Autodesk Inventor part; units mm, degrees
ref_plane "Work Plane2" through (-10, -25.15, 0) normal (0, 1, 0) x (1, 0, 0)
ref_plane "YZ Plane" through (0, 0, 0) normal (1, 0, 0) x (0, 1, 0)
ref_plane "XZ Plane" through (0, 0, 0) normal (0, 1, 0) x (-1, 0, 0)
sketch "Sketch1" plane through (0, 0, 0) normal (0, 0, 1) x (1, 0, 0)
  line L0 (-40, 5) -> (0, 5)
  line L1 (0, 5) -> (0, -5)
  line L2 (0, -5) -> (-40, -5)
  line L3 (-40, -5) -> (-40, 5)
  line L4 (-10, 35) -> (0, 35)
  line L5 (0, 35) -> (0, 5)
  line L6 (0, 5) -> (-10, 5)
  line L7 (-10, 5) -> (-10, 35)
  point P0 (0, 0)
  point P1 (0, 5)
  dimension "d0" = 10
  dimension "d1" = 40
  dimension "d2" = 40
extrude "Extrusion1" add sketch "Sketch1" along normal blind 20
sketch "Sketch2" plane through (-10, 5, 0) normal (-1, 0, 0) x (0, 0, 1)
  line L0 (8.5, 20) -> (11.5, 20) construction
  line L1 (8.5, 17) -> (11.5, 17)
  line L2 (11.5, 23) -> (8.5, 23)
  arc A0 (8.5, 23) -> (8.5, 17) centre (8.5, 20) ccw
  arc A1 (11.5, 17) -> (11.5, 23) centre (11.5, 20) ccw
  line L3 (0, 30) -> (0, 0)
  line L4 (0, 30) -> (20, 30)
  line L5 (10, 21.547) -> (10, 15) construction
  line L6 (11.5, 20) -> (8.5, 20) construction
  line L7 (11.5, 17) -> (8.5, 17)
  line L8 (8.5, 23) -> (11.5, 23)
  arc A2 (11.5, 17) -> (11.5, 23) centre (11.5, 20) ccw
  arc A3 (8.5, 23) -> (8.5, 17) centre (8.5, 20) ccw
  point P0 (0, -5)
  point P1 (10, 20)
  point P2 (10, 18.2735)
  point P3 (10, 30)
  point P4 (10, 20)
  dimension "d5" = 6
  dimension "d6" = 3
  dimension "d7" = 10
  dimension "d8" = 10
extrude "Extrusion2" cut sketch "Sketch2" against normal through all
sketch "Sketch3" plane through (-40, 5, 0) normal (0, 1, 0) x (1, 0, 0)
  line L0 (10, -8.5) -> (10, -11.5) construction
  line L1 (7, -8.5) -> (7, -11.5)
  line L2 (13, -11.5) -> (13, -8.5)
  arc A0 (13, -8.5) -> (7, -8.5) centre (10, -8.5) ccw
  arc A1 (7, -11.5) -> (13, -11.5) centre (10, -11.5) ccw
  line L3 (30, 0) -> (0, 0)
  line L4 (0, 0) -> (0, -20)
  line L5 (15.2557, -10) -> (9.287, -10) construction
  line L6 (10, -11.5) -> (10, -8.5) construction
  line L7 (7, -11.5) -> (7, -8.5)
  line L8 (13, -8.5) -> (13, -11.5)
  arc A2 (7, -11.5) -> (13, -11.5) centre (10, -11.5) ccw
  arc A3 (13, -8.5) -> (7, -8.5) centre (10, -8.5) ccw
  point P0 (40, 0)
  point P1 (10, -10)
  point P2 (12.2713, -10)
  point P3 (0, -10)
  point P4 (10, -10)
  dimension "d11" = 3
  dimension "d12" = 6
  dimension "d13" = 10
  dimension "d14" = 10
extrude "Extrusion3" cut sketch "Sketch3" against normal through all
chamfer "Chamfer1" distance 10 angle 45 1 edges at (-10, 5, 10)
sketch "Sketch10" plane through (0, 0, 20) normal (0, 0, 1) x (1, 0, 0)
  line L0 (-40, -85.3) -> (0, -85.3)
  line L1 (0, -85.3) -> (0, 35)
  line L2 (0, 35) -> (-40, 35)
  line L3 (-40, 35) -> (-40, -85.3)
  line L4 (-40, 5) -> (-40, -5)
  line L5 (0, 35) -> (-10, 35)
  line L6 (0, -5) -> (0, 35)
  line L7 (-40, -5) -> (0, -5)
  line L8 (0, -45.3) -> (19, -45.3)
  line L9 (19, -45.3) -> (19, -5)
  line L10 (19, -5) -> (0, -5)
  line L11 (0, -5) -> (0, -45.3)
  point P0 (0, 0)
  dimension "d30" = 80.3
  dimension "d31" = 120.3
  dimension "d37" = 40.3
  dimension "d38" = 19
extrude "Extrusion7" add sketch "Sketch10" along normal blind 10
ref_plane "Work Plane2" through (-10, -25.15, 0) normal (0, 1, 0) x (1, 0, 0)
mirror "Mirror2" about plane through (-10, -25.15, 0) normal (0, 1, 0) of "Extrusion1", "Extrusion2", "Extrusion3", "Chamfer1"
sketch "Sketch11" plane through (0, 0, 20) normal (0, 0, -1) x (-1, 0, 0)
  line L0 (10, 35) -> (10, 15)
  line L1 (20, 5) -> (10, 15)
  line L2 (20, 5) -> (40, 5)
  line L3 (40, 35) -> (40, 5)
  line L4 (10, 35) -> (40, 35)
  point P0 (0, 0)
extrude "Extrusion8" cut sketch "Sketch11" against normal through all
mirror "Mirror3" about plane through (-10, -25.15, 0) normal (0, 1, 0) of "Extrusion8"
sketch "Sketch12" plane through (0, 0, 20) normal (0, 0, -1) x (-1, 0, 0)
  line L0 (30, -13.5) -> (30, -16.5) construction
  line L1 (27, -13.5) -> (27, -16.5)
  line L2 (33, -16.5) -> (33, -13.5)
  arc A0 (33, -13.5) -> (27, -13.5) centre (30, -13.5) ccw
  arc A1 (27, -16.5) -> (33, -16.5) centre (30, -16.5) ccw
  line L3 (40, -5) -> (40, -45.3)
  line L4 (40, -5) -> (0, -5)
  line L5 (-10, -13.5) -> (-10, -16.5) construction
  line L6 (-13, -13.5) -> (-13, -16.5)
  line L7 (-7, -16.5) -> (-7, -13.5)
  arc A2 (-7, -13.5) -> (-13, -13.5) centre (-10, -13.5) ccw
  arc A3 (-13, -16.5) -> (-7, -16.5) centre (-10, -16.5) ccw
  line L8 (-19, -45.3) -> (-19, -5)
  line L9 (33, -25.15) -> (24.6871, -25.15) construction
  line L10 (30, -36.8) -> (30, -33.8) construction
  line L11 (27, -36.8) -> (27, -33.8)
  line L12 (33, -33.8) -> (33, -36.8)
  arc A4 (27, -36.8) -> (33, -36.8) centre (30, -36.8) ccw
  arc A5 (33, -33.8) -> (27, -33.8) centre (30, -33.8) ccw
  line L13 (-10, -36.8) -> (-10, -33.8) construction
  line L14 (-13, -36.8) -> (-13, -33.8)
  line L15 (-7, -33.8) -> (-7, -36.8)
  arc A6 (-13, -36.8) -> (-7, -36.8) centre (-10, -36.8) ccw
  arc A7 (-7, -33.8) -> (-13, -33.8) centre (-10, -33.8) ccw
  point P0 (0, 0)
  point P1 (30, -15)
  point P2 (-10, -15)
  point P3 (28.8435, -25.15)
  point P4 (40, -25.15)
  point P5 (30, -35.3)
  point P6 (-10, -35.3)
  dimension "d39" = 3
  dimension "d40" = 10
  dimension "d41" = 10
  dimension "d42" = 6
  dimension "d43" = 9
extrude "Extrusion9" cut sketch "Sketch12" against normal through all
fillet "Fillet2" radius 2 3 edges at (-40, 5, 15) (-10, 35, 15) (-10, -85.3, 15)
equation "\"d2\" = d1"
properties part number "0008-10-031 Suport L + placa" material "ABS Plastic"
Source: CAD feature listing. Evaluate the final solid. Frame: model axes, mm. A direction names the side the tool comes from. Give positions to 0.01 mm unless a question says otherwise; leave off trailing zeros. Write each loop counter-clockwise with the first axis right and the second up, starting at its lowest first coordinate (ties: lowest second). Pieces come first, ordered by that corner, then holes. Notation, with made-up numbers: (17, 15.5) -> (69, 15.5) arc R30 cw to (69, 40.5) -> close; hole circle Ø5 at (17, 74). An arc over 180 degrees is marked (long way). Return JSON: item names as keys, results as strings. Group by question number.
1. Section A-A, the plane x = 10. Output: boundary loops of the cut face in (y, z), then the cut area to 3 significant figures.
2. Material intervals for line 1 (Y direction, x = -27.5, z = 15.25); line 2 (X direction, y = -74, z = 26.75); line 3 (Z direction, x = 9.5, y = -25), sorted ascending. Write a range as from..to.
3. Section B-B, the plane z = 9.75. Count the separate pieces of the cut face and the enclosed holes in it, then the cut area to 3 significant figures.
4. Mould query, pull axis Z, two halves, no side actions, for faces 4 (the face through (-27, 0, 10)), 5 (the face through (-20, -45.3, 10)), 6 (the face through (-33, 0, 10)), 7 (the face through (-11, -25, 20)). Classes: +Z half, -Z half, draft (parallel to the pull), parting line (faces both ways), or undercut.
5. Access query for faces 1 (the face through (-5.1, -75.4, 14.5)), 2 (the face through (13, -35, 25)), 3 (the face through (-27, -50, 10)). Directions: +Z, -Z, +X, -X, +Y, -Y. A direction counts if a zero-diameter tool reaches every point of the face in a straight line with its end or side. Return the directions, or none.
6. Pin query (flat end, axial travel): pin 1 Ø3 at (y, z) = (5, 23.5) entering from +X; pin 2 Ø10 at (x, z) = (-25.5, 11.5) entering from +Y; pin 3 Ø8 at (x, z) = (9, 26.5) entering from -Y; pin 4 Ø2 at (x, y) = (-12, 21) entering from -Z. Return the tip coordinate at first contact, or that it passes through.
7. Section D-D, the plane x = -6.5. Output: boundary loops of the cut face in (y, z).
8. Section C-C, the plane y = -32. Output: boundary loops of the cut face in (x, z).
Determined:
{
 "1": {"outline": "(-45.3, 20) -> (-39.8, 20) -> (-39.8, 30) -> (-45.3, 30) -> close; (-30.8, 20) -> (-19.5, 20) -> (-19.5, 30) -> (-30.8, 30) -> close; (-10.5, 20) -> (-5, 20) -> (-5, 30) -> (-10.5, 30) -> close", "area": "223 mm2"},
 "2": {"line 1": "y = -55.3..-45.3, -5..5", "line 2": "x = -10..0", "line 3": "z = 20..30"},
 "3": {"separate pieces": "6", "enclosed holes": "0", "area": "1,260 mm2"},
 "4": {"face 4": "undercut", "face 5": "draft", "face 6": "undercut", "face 7": "-Z half"},
 "5": {"face 1": "+X, -X", "face 2": "+Z, -Z", "face 3": "+Y, -Y"},
 "6": {"pin 1": "stops at x = 0", "pin 2": "stops at y = 5", "pin 3": "stops at y = -45.3", "pin 4": "passes through"},
 "7": {"outline": "(-85.3, 0) -> (-45.3, 0) -> (-45.3, 20) -> (-5, 20) -> (-5, 0) -> (35, 0) -> (35, 30) -> (-85.3, 30) -> close; hole (-78.3, 8.5) arc R3 ccw to (-72.3, 8.5) -> (-72.3, 11.5) arc R3 ccw to (-78.3, 11.5) -> close; hole (22, 8.5) arc R3 ccw to (28, 8.5) -> (28, 11.5) arc R3 ccw to (22, 11.5) -> close"},
 "8": {"outline": "(-40, 20) -> (-32.4, 20) -> (-32.4, 30) -> (-40, 30) -> close; (-27.6, 20) -> (7.6, 20) -> (7.6, 30) -> (-27.6, 30) -> close; (12.4, 20) -> (19, 20) -> (19, 30) -> (12.4, 30) -> close"}
}
